Build history of the part. All positions in model axes, mm. A direction names the side the tool comes from. Round coordinates to 2 decimals unless told otherwise and drop trailing zeros. Order: outer loops, then holes, each group sorted by start corner. A loop starts at its lowest first (then second) coordinate and runs counter-clockwise, first axis right, second up. Notation, with made-up numbers: (45, -4) -> (84, -4) arc R24 ccw to (84, 24) -> close; hole circle Ø10 at (31.25, 28.5). An arc over 180 degrees is marked (long way). Use a Markdown table: item, result. Add a question column.
Item 1: Slice it at C-C, the plane y = 7.5. Give the cut face in (x, z), plus the area to 3 significant figures.
Item 2: Slice it at A-A, the plane y = 40.9. Give the cut face in (x, z).
Item 3: Slice it at D-D, the plane x = 6.35. Give the cut face in (y, z), plus the area to 3 significant figures.
Item 4: Pin check, flat tips, straight feed: pin 1 (5 mm diameter, centred on x = 44.45, z = -6.35, fed in from +Y); pin 2 (9 mm diameter, centred on x = 25.4, y = 25.4, fed in from +Z); pin 3 (2.5 mm diameter, centred on x = 11.98, y = 17.65, fed in from +Z); pin 4 (4.5 mm diameter, centred on x = 29, y = 23.5, fed in from -Z). Stop position of each tip, or through.
Item 5: Two-plate mould, pull along Z, no slides. Class faces 4 (the face through (25, 50.8, -6)), 5 (the face through (26, 22, -6.35)), 6 (the face through (7.856, 6.261, -3.454)): released by +Z, released by -Z, zero draft, split by the parting line, or undercut.
Item 6: 3-axis set-ups, long thin cutter, end or side, ignore diameter. For faces 1 (the face through (7.856, 44.539, -3.454)), 2 (the face through (44, 12.7, -6)), 3 (the face through (23, 28, -4.762)): which of +Z, -Z, +X, -X, +Y, -Y reach the whole face in a straight line?
Item 7: Slice it at B-B, the plane z = -1.25. Give the cut face in (x, y) (3 decimals).
Item 8: Probe L1, parallel to Y at x = 12, z = -11.5; L2, parallel to X at y = 46, z = -6.35; L3, parallel to Z at x = 44.45, y = 48. List the from-to ranges inside material, lowest first.
from build123d import *

# Parameters (mm, degrees)
SKETCH1_W           = 50.8
SKETCH1_H           = 12.7
BOSS_EXTRUDE1_DEPTH = 50.8
SKETCH2_R           = 3.175
CUT_EXTRUDE1_DEPTH  = 13.7
SKETCH3_R           = 9.525
CUT_EXTRUDE2_DEPTH  = 4.7625
SKETCH4_R           = 3.2639
CUT_EXTRUDE3_DEPTH  = 12.7
SKETCH5_R           = 1.65
CUT_EXTRUDE4_DEPTH  = 13.7
SKETCH6_R           = 7.62
CUT_EXTRUDE5_DEPTH  = 6.35


with BuildPart() as part:
    # Sketch1 → Boss-Extrude1 (new body)
    with BuildSketch(Plane(origin=(0, 0, 0), x_dir=(1, 0, 0), z_dir=(0, 1, 0))):
        with Locations((25.4, 6.35)):
            Rectangle(SKETCH1_W, SKETCH1_H)
    extrude(amount=BOSS_EXTRUDE1_DEPTH)

    # Sketch2 → Cut-Extrude1 (cut, through all)
    with BuildSketch(Plane.XY):
        with Locations((25.4, 25.4)):
            Circle(SKETCH2_R)
    extrude(amount=-CUT_EXTRUDE1_DEPTH, mode=Mode.SUBTRACT)

    # Sketch3 → Cut-Extrude2 (cut)
    with BuildSketch(Plane.XY):
        with Locations((25.4, 25.4)):
            Circle(SKETCH3_R)
    extrude(amount=-CUT_EXTRUDE2_DEPTH, mode=Mode.SUBTRACT)

    # Sketch4 → Cut-Extrude3 (cut)
    with BuildSketch(Plane(origin=(0, 50.8, 0), x_dir=(1, 0, 0), z_dir=(0, 1, 0))):
        with Locations((6.35, 6.35)):
            Circle(SKETCH4_R)
        with Locations((44.45, 6.35)):
            Circle(SKETCH4_R)
    cut_extrude3 = extrude(amount=-CUT_EXTRUDE3_DEPTH, mode=Mode.SUBTRACT)

    # Mirror1: Cut-Extrude3 across plane
    add(cut_extrude3.mirror(Plane.ZX.offset(25.4)), mode=Mode.SUBTRACT)

    # Sketch5 → Cut-Extrude4 (cut, through all)
    with BuildSketch(Plane.XY):
        with Locations((25.4, 40.9)):
            Circle(SKETCH5_R)
        with Locations((38.823393759, 33.15)):
            Circle(SKETCH5_R)
        with Locations((38.823393759, 17.65)):
            Circle(SKETCH5_R)
        with Locations((25.4, 9.9)):
            Circle(SKETCH5_R)
        with Locations((11.976606241, 17.65)):
            Circle(SKETCH5_R)
        with Locations((11.976606241, 33.15)):
            Circle(SKETCH5_R)
    extrude(amount=-CUT_EXTRUDE4_DEPTH, mode=Mode.SUBTRACT)

    # Sketch6 → Cut-Extrude5 (cut)
    with BuildSketch(Plane(origin=(0, 0, -12.7), x_dir=(-1, 0, 0), z_dir=(0, 0, -1))):
        with Locations((-25.4, 25.4)):
            Circle(SKETCH6_R)
    extrude(amount=-CUT_EXTRUDE5_DEPTH, mode=Mode.SUBTRACT)


solid = part.part
Check sheet entries:
| question | item | result |
|---|---|---|
| 1 | outline | (0, -12.7) -> (50.8, -12.7) -> (50.8, 0) -> (0, 0) -> close; hole circle Ø6.53 at (6.35, -6.35); hole circle Ø6.53 at (44.45, -6.35) |
| 1 | area | 578 mm2 |
| 2 | outline | (0, -12.7) -> (23.75, -12.7) -> (23.75, 0) -> (0, 0) -> close; (27.05, -12.7) -> (50.8, -12.7) -> (50.8, 0) -> (27.05, 0) -> close; hole circle Ø6.53 at (6.35, -6.35); hole circle Ø6.53 at (44.45, -6.35) |
| 3 | outline | (0, -12.7) -> (50.8, -12.7) -> (50.8, -9.61) -> (38.1, -9.61) -> (38.1, -3.09) -> (50.8, -3.09) -> (50.8, 0) -> (0, 0) -> (0, -3.09) -> (12.7, -3.09) -> (12.7, -9.61) -> (0, -9.61) -> close |
| 3 | area | 479 mm2 |
| 4 | pin 1 | y = 38.1 |
| 4 | pin 2 | z = -4.76 |
| 4 | pin 3 | through |
| 4 | pin 4 | z = -6.35 |
| 5 | face 4 | zero draft |
| 5 | face 5 | released by -Z |
| 5 | face 6 | undercut |
| 6 | face 1 | +Y |
| 6 | face 2 | -Y |
| 6 | face 3 | +Z |
| 7 | outline | (0, 0) -> (50.8, 0) -> (50.8, 50.8) -> (0, 50.8) -> close; hole circle Ø3.3 at (11.977, 17.65); hole circle Ø3.3 at (11.977, 33.15); hole circle Ø19.05 at (25.4, 25.4); hole circle Ø3.3 at (25.4, 9.9); hole circle Ø3.3 at (25.4, 40.9); hole circle Ø3.3 at (38.823, 17.65); hole circle Ø3.3 at (38.823, 33.15) |
| 8 | L1 | 0 to 16, 19.3 to 31.5, 34.8 to 50.8 |
| 8 | L2 | 0 to 3.09, 9.61 to 41.19, 47.71 to 50.8 |
| 8 | L3 | -12.7 to -9.61, -3.09 to 0 |
